Can you work these out from the model? Positions are in its coordinate system, mm. A direction names the side the tool comes from. Round coordinates to 2 decimals unless told otherwise and drop trailing zeros. Write each loop counter-clockwise with the first axis right and the second up, starting at its lowest first coordinate (ties: lowest second). Pieces come first, ordered by that corner, then holes. Notation, with made-up numbers: M 28.5,23 L 47.5,23 A16 cw 47.5,29 Z; hole C 51,-10.5 d7. An arc over 180 degrees is marked long. Answer in a Markdown table with one row per item. Add a question column.
(1) Suppose I cut it at B-B, the plane y = 5.08. Write out the boundary of the cut face in (x, z) (1 decimal), then the cut area to 3 significant figures.
(2) If I drill on probe 1 along Y at (x, z) = (7.75, -17); probe 2 along Z at (x, y) = (8.25, 7.5) (3 decimals); probe 3 along Z at (x, y) = (7.5, 8.5) (3 decimals), over which ranges is the centre line in solid material (lowest first)?
(3) Suppose I cut it at D-D, the plane y = 1. Write out the boundary of the cut face in (x, z) (1 decimal).
(4) For faces 4 (the face through (7, 5, -2.184)), 5 (the face through (2, 10.16, 18)), 6 (the face through (2, 0, 18)), which set-ups out of +Z, -Z, +X, -X, +Y, -Y let a thin tool reach every point of the face, with its end or its side?
(5) Suppose I cut it at C-C, the plane z = 15.5. Write out the boundary of the cut face in (x, y).
(6) I'm going to push flat-ended pins straight in: pin 1 (5.5 mm diameter, centred on x = 6.62, z = -24.27, fed in from -Y); pin 2 (6 mm diameter, centred on y = 4, z = -18.5, fed in from -X); pin 3 (3 mm diameter, centred on y = 3.5, z = 23, fed in from +X); pin 4 (1.4 mm diameter, centred on x = 4.5, y = 4.5, fed in from -Z). Where does each tip first touch, or does it pass through?
(7) Suppose I cut it at A-A, the plane x = 2.25. Count the separate pieces of the cut face and the enclosed holes in it, then the cut area to 3 significant figures.
(8) If we mould it in two halves opening along Y, with no side actions, what happens to faces 1 (the face through (7, 6.817, -17)), 2 (the face through (7, 11.748, -15)), 3 (the face through (6.751, 9.248, -9.263))? For each: released by +Y, released by -Y, zero draft, split by the parting line, or undercut.
from build123d import *

# Parameters (mm, degrees)
SKETCH1_W                = 4.7625
SKETCH1_H                = 34.798
BOSS_EXTRUDE1_DEPTH      = 10.16
SKETCH2_R                = 2.54
CUT_EXTRUDE1_DEPTH       = 37.562382448
BOSS_EXTRUDE2_DEPTH      = 6.6675
BOSS_EXTRUDE2_DEPTH_BACK = 7.5565
SKETCH3_W                = 13.23848
SKETCH3_H                = 34.0614
SKETCH3_R                = 2.99974
SKETCH6_W                = 13.23848
SKETCH6_H                = 4.5085
CUT_EXTRUDE3_DEPTH       = 28.702
FILLET1_R                = 2.54
FILLET2_R                = 1.27


with BuildPart() as part:
    # Sketch1 → Boss-Extrude1 (new body)
    with BuildSketch(Plane(origin=(0, 0, 0), x_dir=(1, 0, 0), z_dir=(0, 1, 0))):
        with Locations((2.38125, -17.399)):
            Rectangle(SKETCH1_W, SKETCH1_H)
    extrude(amount=BOSS_EXTRUDE1_DEPTH)

    # Sketch2 → Cut-Extrude1 (cut, through all)
    with BuildSketch(Plane(origin=(4.7625, 0, 0), x_dir=(0, 0, -1), z_dir=(1, 0, 0))):
        with Locations((-27.178, 5.08)):
            Circle(SKETCH2_R)
        with Locations((-14.478, 5.08)):
            Circle(SKETCH2_R)
    extrude(amount=-CUT_EXTRUDE1_DEPTH, mode=Mode.SUBTRACT)

    # Sketch3 → Boss-Extrude2 (add, two sides: drawn at the far end of the back side and taken through both)
    with BuildSketch(Plane(origin=(0, 5.08, 0), x_dir=(1, 0, 0), z_dir=(0, 1, 0)).offset(-BOSS_EXTRUDE2_DEPTH_BACK)):
        with Locations((6.61924, 13.8557)):
            Rectangle(SKETCH3_W, SKETCH3_H)
        with Locations(Location((6.61924, 6.26618, 0), (0, 0, 270))):
            Circle(SKETCH3_R, mode=Mode.SUBTRACT)
        with Locations(Location((6.61924, 24.26716, 0), (0, 0, 270))):
            Circle(SKETCH3_R, mode=Mode.SUBTRACT)
    extrude(amount=BOSS_EXTRUDE2_DEPTH + BOSS_EXTRUDE2_DEPTH_BACK)

    # Sketch6 → Cut-Extrude3 (cut)
    with BuildSketch(Plane(origin=(0, 0, -30.8864), x_dir=(-1, 0, 0), z_dir=(0, 0, -1))):
        with Locations((-6.61924, 4.56311)):
            Rectangle(SKETCH6_W, SKETCH6_H)
    extrude(amount=-CUT_EXTRUDE3_DEPTH, mode=Mode.SUBTRACT)

    # Fillet1
    fillet1_edges = [part.edges().sort_by_distance(p)[0] for p in [
        (4.7625, 5.08, 3.175),
        (13.23848, -0.08382, -30.8864),
        (13.23848, 9.28243, -30.8864),
        (2.38125, 0, 34.798),
        (2.38125, 10.16, 34.798),
    ]]
    fillet(fillet1_edges, radius=FILLET1_R)

    # Fillet2
    fillet2_edges = [part.edges().sort_by_distance(p)[0] for p in [
        (6.61924, -2.4765, 3.175),
        (13.23848, 4.6355, 3.175),
        (6.61924, 11.7475, 3.175),
    ]]
    fillet(fillet2_edges, radius=FILLET2_R)


solid = part.part
Calculated:
| question | item | result |
|---|---|---|
| 1 | outline | M 0,-2.2 L 13.2,-2.2 L 13.2,1.9 A1.3 ccw 12,3.2 L 7.3,3.2 A2.5 cw 4.8,5.7 L 4.8,11.9 L 0,11.9 Z; M 0,17 L 4.8,17 L 4.8,24.6 L 0,24.6 Z; M 0,29.7 L 4.8,29.7 L 4.8,34.8 L 0,34.8 Z |
| 1 | area | 174 mm² |
| 2 | probe 1 | -2.48 to 2.31, 6.82 to 11.75 |
| 2 | probe 2 | -30.886 to -26.785, -21.749 to -8.784, -3.748 to 3.175 |
| 2 | probe 3 | -30.886 to -27.135, -21.4 to -9.134, -3.399 to 3.175 |
| 3 | outline | M 0,-30.9 L 10.7,-30.9 A2.5 ccw 13.2,-28.3 L 13.2,1.9 A1.3 ccw 12,3.2 L 7.3,3.2 A2.5 cw 4.8,5.7 L 4.8,34.3 L 0,34.3 Z; hole C 6.6,-24.3 d6; hole C 6.6,-6.3 d6 |
| 4 | face 4 | -Z, +X, -X |
| 4 | face 5 | +Z, +X, -X, +Y |
| 4 | face 6 | +Z, +X, -X, -Y |
| 5 | outline | M 0,0 L 4.76,0 L 4.76,2.75 L 0,2.75 Z; M 0,7.41 L 4.76,7.41 L 4.76,10.16 L 0,10.16 Z |
| 6 | pin 1 | through |
| 6 | pin 2 | x = 0 |
| 6 | pin 3 | x = 4.76 |
| 6 | pin 4 | z = -2.18 |
| 7 | separate pieces | 1 |
| 7 | enclosed holes | 2 |
| 7 | area | 632 mm² |
| 8 | face 1 | undercut |
| 8 | face 2 | released by +Y |
| 8 | face 3 | zero draft |
